Answer from the drawing. Dimensions are ordinates in mm from the lowest x, y and z of the part. Round coordinates to 2 decimals unless told otherwise and drop trailing zeros. Loops run counter-clockwise (first coordinate to the right, second up) from the corner with the lowest first, then second, coordinate; pieces in that order, holes last. Notation, with made-up numbers: (-12.5, 68) - (45.5, 68) arc R22 ccw to (45.5, 91) - close; hole circle Ø5 at (-15.5, 86). An arc over 180 degrees is marked (long way). Answer as CSV lines item,"result".
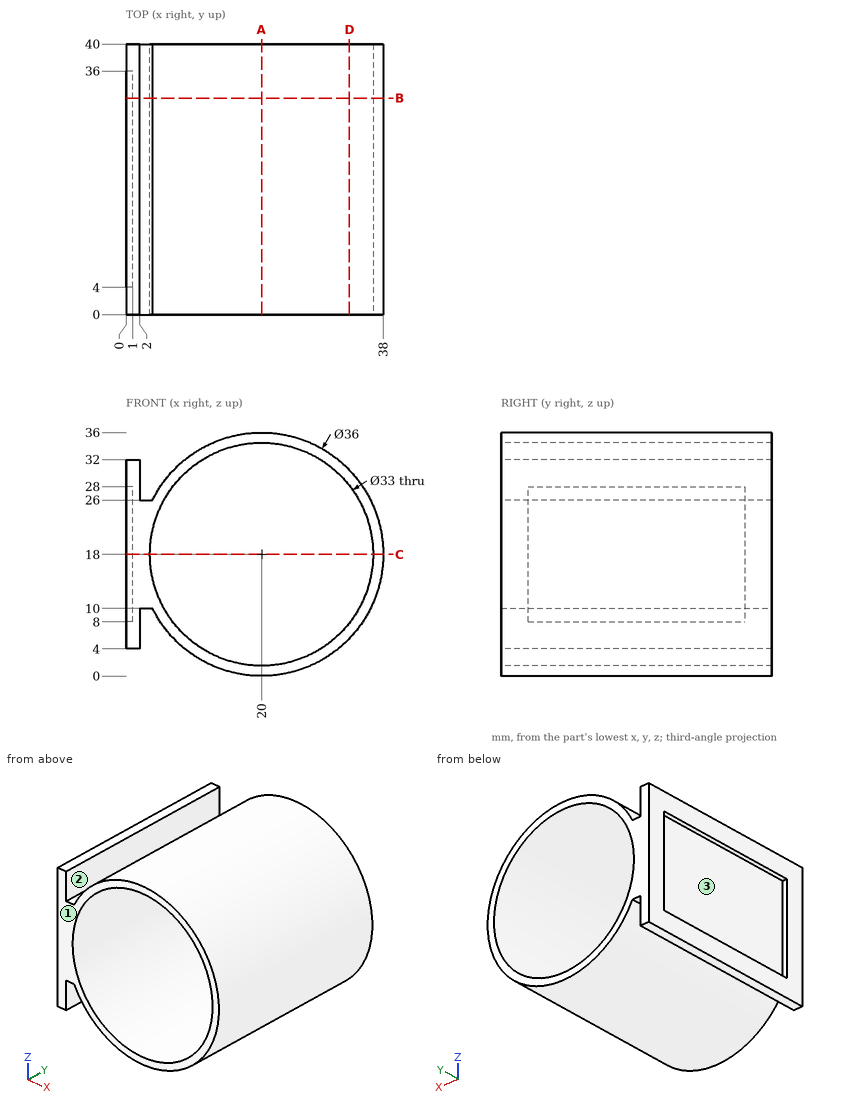
1) A cutting plane is placed at C-C, the plane z = 18. Determine the outline of the cut face in (x, y), plus the area to 3 significant figures.
Entries:
outline,"(0, 0) - (3.5, 0) - (3.5, 40) - (0, 40) - (0, 36) - (1, 36) - (1, 4) - (0, 4) - close; (36.5, 0) - (38, 0) - (38, 40) - (36.5, 40) - close"
area,"168 mm^2"
2) A cutting plane is placed at A-A, the plane x = 20. Determine the outline of the cut face in (y, z).
Entries:
outline,"(0, 0) - (40, 0) - (40, 1.5) - (0, 1.5) - close; (0, 34.5) - (40, 34.5) - (40, 36) - (0, 36) - close"
3) A cutting plane is placed at D-D, the plane x = 33. Determine the outline of the cut face in (y, z), plus the area to 3 significant figures.
Entries:
outline,"(0, 5.55) - (40, 5.55) - (40, 7.84) - (0, 7.84) - close; (0, 28.16) - (40, 28.16) - (40, 30.45) - (0, 30.45) - close"
area,"183 mm^2"
4) A cutting plane is placed at B-B, the plane y = 32. Determine the outline of the cut face in (x, z).
Entries:
outline,"(0, 4) - (2, 4) - (2, 10) - (3.88, 10) arc R18 ccw (long way) to (3.88, 26) - (2, 26) - (2, 32) - (0, 32) - (0, 28) - (1, 28) - (1, 8) - (0, 8) - close; hole circle Ø33 at (20, 18)"
5) Each of these flat-tipped pins is pushed along its axis until it touches: P1, Ø3, axis at y = 24.5, z = 29.5, coming from the +X side; P2, Ø2, axis at x = 1.5, y = 20, coming from the -Z side; P3, Ø10, axis at y = 34.5, z = 28, coming from the +X side; P4, Ø20, axis at x = 20, z = 18, coming from the -Y side. Where does it stop, or does it pass through?
Entries:
P1,"stops at x = 34.97"
P2,"stops at z = 4"
P3,"stops at x = 37.29"
P4,"passes through"
6) Find the intervals of material crossed by line 1 (Z direction, x = 20, y = 16.5); line 2 (X direction, y = 25, z = 6); line 3 (X direction, y = 31, z = 29), in increasing order.
Entries:
line 1,"z = 0 to 1.5, 34.5 to 36"
line 2,"x = 0 to 2, 6.58 to 8.68, 31.32 to 33.42"
line 3,"x = 0 to 2, 5.75 to 7.7, 32.3 to 34.25"
7) The mould has two halves that part along Y. Classify the marked faces 1, 2 and 3: pulls with the +Y half, pulls with the -Y half, needs draft (parallel to the pull), parting line crosses it, or undercut.
Entries:
face 1,"pulls with the -Y half"
face 2,"needs draft"
face 3,"undercut"
